Autodesk Inventor part; units mm, degrees
ref_plane "YZ Plane" through (0, 0, 0) normal (1, 0, 0) x (0, 1, 0)
ref_plane "XZ Plane" through (0, 0, 0) normal (0, 1, 0) x (-1, 0, 0)
ref_plane "XY Plane" through (0, 0, 0) normal (0, 0, 1) x (1, 0, 0)
sketch "Sketch1" plane through (0, 0, 0) normal (0, 0, 1) x (1, 0, 0)
  line L0 (0, 0) -> (-25.4, 0)
  line L1 (-25.4, 0) -> (-25.4, 50.8)
  line L2 (-25.4, 50.8) -> (0, 50.8)
  line L3 (0, 50.8) -> (0, 0)
  line L4 (-22.225, 3.175) -> (-3.175, 3.175)
  line L5 (-3.175, 3.175) -> (-3.175, 47.625)
  line L6 (-3.175, 47.625) -> (-22.225, 47.625)
  line L7 (-22.225, 47.625) -> (-22.225, 3.175)
  dimension "d0" = 25.4
  dimension "d1" = 50.8
  dimension "d2" = 3.175
extrude "Extrusion1" add sketch "Sketch1" along normal blind 762
sketch "Sketch2" plane through (0, 0, 0) normal (1, 0, 0) x (0, 0, -1)
  circle A0 centre (-50.8, 25.4) radius 14.2875
  line L0 (0, 50.8) -> (0, 0)
  line L1 (0, 0) -> (-762, 0)
  dimension "d5" = 50.8
  dimension "d6" = 25.4
  dimension "d7" = 28.575
extrude "Extrusion2" cut sketch "Sketch2" against normal blind 930.1395
sketch "Sketch3" plane through (0, 0, 0) normal (1, 0, 0) x (0, 0, -1)
  circle A0 centre (-723.9, 25.4) radius 14.2875
  line L0 (-762, 0) -> (-762, 50.8)
  line L1 (0, 50.8) -> (-762, 50.8)
  point P0 (0, 0)
  dimension "d10" = 38.1
  dimension "d11" = 25.4
  dimension "d12" = 28.575
extrude "Extrusion3" cut sketch "Sketch3" against normal blind 25.4
properties part number "DRL Angle"
Here's how the part is built. I have some questions about the finished solid (model axes, mm). A direction names the side the tool comes from. Round coordinates to 2 decimals unless told otherwise and drop trailing zeros. Write each loop counter-clockwise with the first axis right and the second up, starting at its lowest first coordinate (ties: lowest second). Pieces come first, ordered by that corner, then holes.
1. If we mould it in two halves opening along Y, with no side actions, what happens to faces 1 (the cylindrical face through (-1.565, 26.028, 738.174)), 2 (the flat face through (-13, 3.175, 376)), 3 (the flat face through (-13, 50.8, 376)), 4 (the flat face through (-13, 0, 376))? For each: released by +Y, released by -Y, zero draft, split by the parting line, or undercut.
2. For faces 5 (the flat face through (-22.225, 26, 376)), 6 (the cylindrical face through (-23.79, 26.028, 65.074)), which set-ups out of +Z, -Z, +X, -X, +Y, -Y let a thin tool reach every point of the face, with its end or its side?
3. Suppose I cut it at C-C (z = 117.5). List the corners of the cut face in (x, y) for me (3 decimals), and give its area (3 significant figures).
4. Suppose I cut it at D-D (y = 25.4). List the corners of the cut face in (x, z) for me (1 decimal).
5. I need wall thicknesses on L1, parallel to X at y = 31.5, z = 619 (3 decimals); L2, parallel to Y at x = -24.45, z = 50.8; L3, parallel to Z at x = -0.75, y = 21.5. Which ranges of each line are inside material? Lowest first, please.
6. Will this pin go through, and if not, where does the flat tip stop? pin 1 Ø23 at (y, z) = (25.4, 723.9) entering from -X.
7. Suppose I cut it at A-A (z = 723.9). List the corners of the cut face in (x, y) for me (1 decimal).
8. Suppose I cut it at B-B (x = -17.5). List the corners of the cut face in (y, z) for me (3 decimals).
Answer sheet:
1. face 1: undercut
1. face 2: undercut
1. face 3: released by +Y
1. face 4: released by -Y
2. face 5: +Z, -Z
2. face 6: +X, -X
3. outline: (-25.4, 0) - (0, 0) - (0, 50.8) - (-25.4, 50.8) - close; hole (-22.225, 3.175) - (-3.175, 3.175) - (-3.175, 47.625) - (-22.225, 47.625) - close
3. area: 444 mm2
4. outline: (-25.4, 0) - (-22.2, 0) - (-22.2, 36.5) - (-25.4, 36.5) - close; (-25.4, 65.1) - (-22.2, 65.1) - (-22.2, 709.6) - (-25.4, 709.6) - close; (-25.4, 738.2) - (-22.2, 738.2) - (-22.2, 762) - (-25.4, 762) - close; (-3.2, 0) - (0, 0) - (0, 36.5) - (-3.2, 36.5) - close; (-3.2, 65.1) - (0, 65.1) - (0, 709.6) - (-3.2, 709.6) - close; (-3.2, 738.2) - (0, 738.2) - (0, 762) - (-3.2, 762) - close
5. L1: x = -25.4 to -22.225, -3.175 to 0
5. L2: y = 0 to 11.11, 39.69 to 50.8
5. L3: z = 0 to 37.06, 64.54 to 710.16, 737.64 to 762
6. pin 1: passes through
7. outline: (-25.4, 0) - (0, 0) - (0, 11.1) - (-3.2, 11.1) - (-3.2, 3.2) - (-22.2, 3.2) - (-22.2, 11.1) - (-25.4, 11.1) - close; (-25.4, 39.7) - (-22.2, 39.7) - (-22.2, 47.6) - (-3.2, 47.6) - (-3.2, 39.7) - (0, 39.7) - (0, 50.8) - (-25.4, 50.8) - close
8. outline: (0, 0) - (3.175, 0) - (3.175, 762) - (0, 762) - close; (47.625, 0) - (50.8, 0) - (50.8, 762) - (47.625, 762) - close
